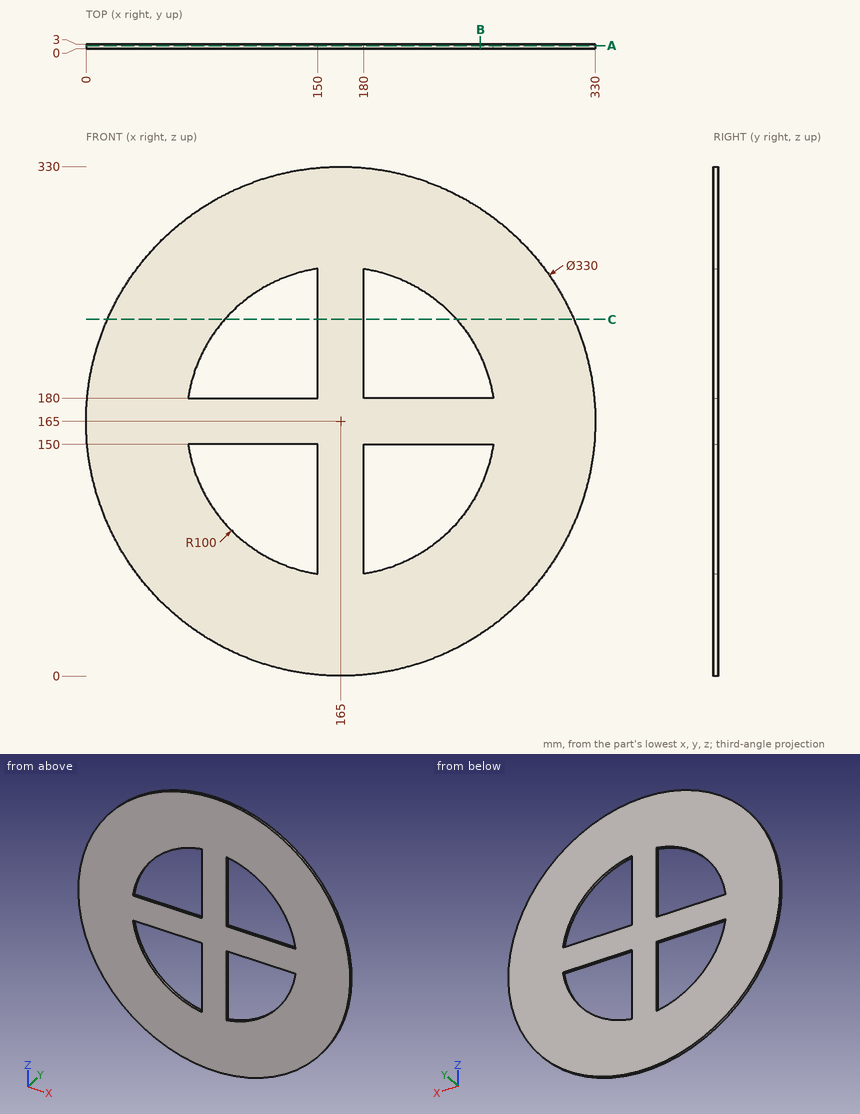
Part print with two shaded views. Sizes in mm from the minimum x, y, z corner. Round coordinates to 2 decimals unless told otherwise and drop trailing zeros. Loops run counter-clockwise (first coordinate to the right, second up) from the corner with the lowest first, then second, coordinate; pieces in that order, holes last. Notation, with made-up numbers: M 31,-4.5 L 79,-4.5 A20 cw 79,7.5 Z; hole C 74,6 d8. An arc over 180 degrees is marked long. Return JSON: item names as keys, results as strings. Group by question number.
(1) Wall check: probe 1 along X at (y, z) = (0.3, 107); probe 2 along Z at (x, y) = (210.5, 2.8); probe 3 along X at (y, z) = (2.95, 127.5). Give the ranges that are in metal, low to high. Write a range as [from, to].
(2) Drop flat-ended pins along their axis: P1, Ø1.5, axis at y = 1.5, z = 106, coming from the -X side; P2, Ø1.5, axis at y = 2.5, z = 188.5, coming from the -X side; P3, Ø0.9, axis at y = 1, z = 220.5, coming from the +X side. Give the stop position or say it passes through.
(3) Saw through at A-A, the plane y = 1.95. List the corners of the cut face in (x, z), and give its area (3 significant figures).
(4) Saw through at C-C, the plane z = 231. List the corners of the cut face in (x, y) (3 decimals).
(5) Saw through at B-B, the plane x = 255.5. List the corners of the cut face in (y, z).
Answer list:
{
 "1": {"probe 1": "[10.53, 83.54], [150, 180], [246.46, 319.47]", "probe 2": "[6.4, 75.95], [150, 180], [254.05, 323.6]", "probe 3": "[4.32, 72.3], [150, 180], [257.7, 325.68]"},
 "2": {"P1": "x = 10.62", "P2": "x = 1.58", "P3": "x = 320.55"},
 "3": {"outline": "C 165,165 d330; hole M 66.13,150 A100 ccw 150,66.13 L 150,150 Z; hole M 66.13,180 L 150,180 L 150,263.87 A100 ccw Z; hole M 180,66.13 A100 ccw 263.87,150 L 180,150 Z; hole M 180,180 L 263.87,180 A100 ccw 180,263.87 Z", "area": "65,200 mm2"},
 "4": {"outline": "M 13.775,0 L 89.873,0 L 89.873,3 L 13.775,3 Z; M 150,0 L 180,0 L 180,3 L 150,3 Z; M 240.127,0 L 316.225,0 L 316.225,3 L 240.127,3 Z"},
 "5": {"outline": "M 0,27.03 L 3,27.03 L 3,122.46 L 0,122.46 Z; M 0,150 L 3,150 L 3,180 L 0,180 Z; M 0,207.54 L 3,207.54 L 3,302.97 L 0,302.97 Z"}
}
